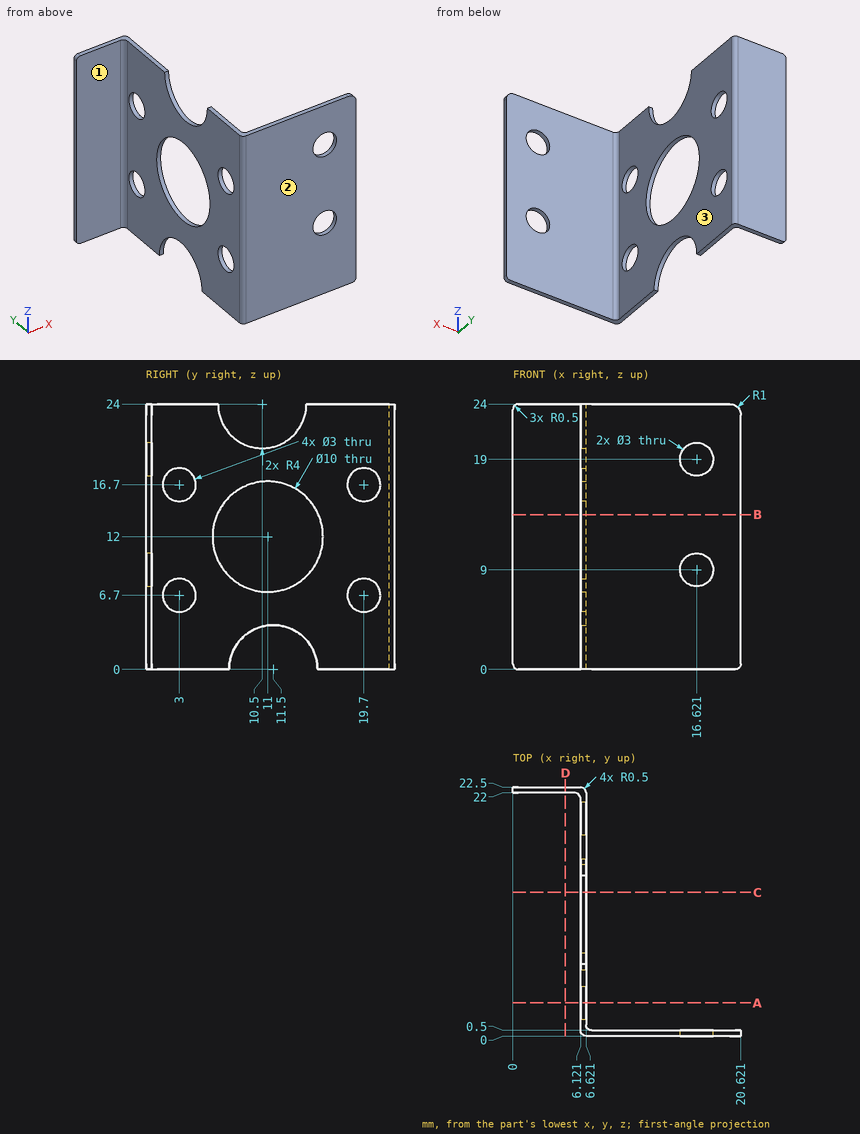
Part print with two shaded views. Sizes in mm from the minimum x, y, z corner. A direction names the side the tool comes from. Give positions to 0.01 mm unless a question says otherwise; leave off trailing zeros. Write each loop counter-clockwise with the first axis right and the second up, starting at its lowest first coordinate (ties: lowest second). Pieces come first, ordered by that corner, then holes.
1) Cut at B-B on z = 14. Write the cut outline in (x, y), then the cut area to 3 significant figures.
Resolved:
outline: (0, 22) - (5.62, 22) arc R0.5 cw to (6.12, 21.5) - (6.12, 15.58) - (6.62, 15.58) - (6.62, 22) arc R0.5 ccw to (6.12, 22.5) - (0, 22.5) - close; (6.12, 0.5) arc R0.5 ccw to (6.62, 0) - (20.62, 0) - (20.62, 0.5) - (7.12, 0.5) arc R0.5 cw to (6.62, 1) - (6.62, 6.42) - (6.12, 6.42) - close
area: 16.7 mm2
2) Probe L1, parallel to Y at x = 6.4, z = 6.7 (1 decimal); L2, parallel to Y at x = 6.55, z = 6.7 (3 decimals); L3, parallel to Y at x = 16, z = 2.25. List the from-to ranges inside material, lowest first.
Resolved:
L1: y = 0.1 to 1.5, 4.5 to 18.2, 21.2 to 22.4
L2: y = 0.005 to 1.5, 4.5 to 18.2, 21.2 to 22.257
L3: y = 0 to 0.5
3) Cut at A-A on y = 3. Write the cut outline in (x, z).
Resolved:
outline: (6.12, 0) - (6.62, 0) - (6.62, 5.2) - (6.12, 5.2) - close; (6.12, 8.2) - (6.62, 8.2) - (6.62, 15.2) - (6.12, 15.2) - close; (6.12, 18.2) - (6.62, 18.2) - (6.62, 24) - (6.12, 24) - close
4) Cut at C-C on y = 13. Write the cut outline in (x, z), then the cut area to 3 significant figures.
Resolved:
outline: (6.12, 3.71) - (6.62, 3.71) - (6.62, 7.42) - (6.12, 7.42) - close; (6.12, 16.58) - (6.62, 16.58) - (6.62, 20.88) - (6.12, 20.88) - close
area: 4.00 mm2
5) Which spindle directions (+Z, -Z, +X, -X, +Y, -Y) get a long thin tool onto all of the face, cutting with end or side? Do the marked faces 1, 2 and 3. Say none if no direction does.
Resolved:
face 1: +Z, -Z, -X, -Y
face 2: +Z, -Z, +X, -X, -Y
face 3: +Z, -Z, +X, +Y
6) Cut at D-D on x = 4.75. Write the cut outline in (y, z).
Resolved:
outline: (22, 0) - (22.5, 0) - (22.5, 24) - (22, 24) - close
7) Pin check, flat tips, straight feed: pin 1 (5 mm diameter, centred on y = 18.5, z = 18.5, fed in from -X); pin 2 (3 mm diameter, centred on x = 6, y = 11, fed in from +Z); pin 3 (4.5 mm diameter, centred on x = 2, z = 7.5, fed in from -Y). Stop position of each tip, or through.
Resolved:
pin 1: stops at x = 6.12
pin 2: stops at z = 20.53
pin 3: stops at y = 22
